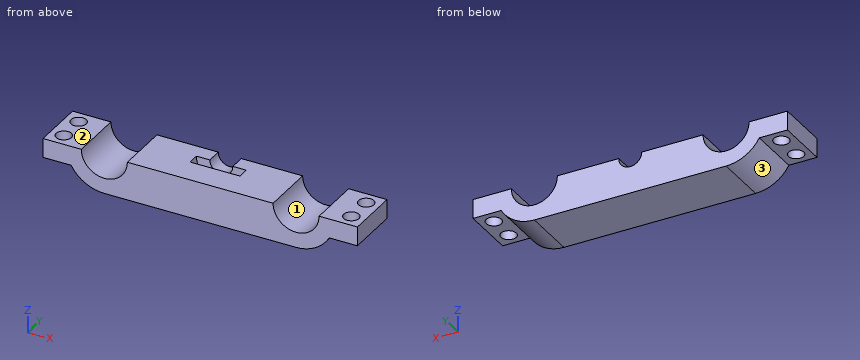
```python
from build123d import *

# Parameters (mm, degrees)
BOSS_EXTRUDE1_DEPTH     = 14
CUT_EXTRUDE1_DEPTH      = 45.463468151
CUT_EXTRUDE1_DEPTH_BACK = 45.463468151
SKETCH4_R               = 2
SKETCH5_W               = 9.30871577
SKETCH5_H               = 4.044371358
BOSS_EXTRUDE2_DEPTH     = 7
CUT_EXTRUDE2_START      = 1.5
SKETCH6_R               = 6.5
CUT_EXTRUDE2_DEPTH      = 1.5


with BuildPart() as part:
    # Sketch2 → Boss-Extrude1 (new body)
    with BuildSketch(Plane(origin=(0, 0, 0), x_dir=(1, 0, 0), z_dir=(0, 1, 0))):
        with BuildLine():
            Line((-3, 0), (-19, 0))
            ThreePointArc((-19, 0), (-25, 6), (-31, 0))
            Line((-31, 0), (-41, 0))
            Line((-41, 0), (-41, 5))
            Line((-41, 5), (-33.660254038, 5))
            ThreePointArc((-33.660254038, 5), (-30, 8.660254038), (-25, 10))
            Line((-25, 10), (25, 10))
            ThreePointArc((25, 10), (30, 8.660254038), (33.660254038, 5))
            Line((33.660254038, 5), (41, 5))
            Line((41, 5), (41, 0))
            Line((41, 0), (31, 0))
            ThreePointArc((31, 0), (25, 6), (19, 0))
            Line((19, 0), (3, 0))
            ThreePointArc((3, 0), (0, 3), (-3, 0))
        make_face()
    extrude(amount=BOSS_EXTRUDE1_DEPTH)

    # Sketch4 → Cut-Extrude1 (cut, two sides: drawn at the far end of the back side and taken through both)
    with BuildSketch(Plane.XY.offset(-CUT_EXTRUDE1_DEPTH_BACK)):
        with Locations((-37.5, 10.5)):
            Circle(SKETCH4_R)
        with Locations((-37.5, 3.5)):
            Circle(SKETCH4_R)
        with Locations((37.5, 10.5)):
            Circle(SKETCH4_R)
        with Locations((37.5, 3.5)):
            Circle(SKETCH4_R)
    extrude(amount=CUT_EXTRUDE1_DEPTH + CUT_EXTRUDE1_DEPTH_BACK, mode=Mode.SUBTRACT)

    # Sketch5 → Boss-Extrude2 (add)
    with BuildSketch(Plane.XZ):
        with Locations((-0.028958253, -2.022185679)):
            Rectangle(SKETCH5_W, SKETCH5_H)
    extrude(amount=-BOSS_EXTRUDE2_DEPTH)

    # Sketch6 → Cut-Extrude2 (cut, symmetric)
    with BuildSketch(Plane(origin=(0, 7, 0), x_dir=(1, 0, 0), z_dir=(0, 1, 0)).offset(CUT_EXTRUDE2_START)):
        Circle(SKETCH6_R)
    extrude(amount=CUT_EXTRUDE2_DEPTH, both=True, mode=Mode.SUBTRACT)


solid = part.part
```
Here's how the part is built. I have some questions about the finished solid (model axes, mm). Face numbers are marked on the shaded views. Round coordinates to 2 decimals unless told otherwise and drop trailing zeros. Order: outer loops, then holes, each group sorted by start corner. A loop starts at its lowest first (then second) coordinate and runs counter-clockwise, first axis right, second up. Notation, with made-up numbers: (-37, 87) -> (4, 87) arc R22 cw to (4, 111) -> close; hole circle Ø11 at (32, 9). An arc over 180 degrees is marked (long way). Use a Markdown table: item, result. Add a question column.
(1) If we mould it in two halves opening along X, with no side actions, what happens to the marked faces 1, 2 and 3? For each: released by +X, released by -X, zero draft, split by the parting line, or undercut.
(2) Suppose I cut it at A-A, the plane y = 3.5. Please give me the cut outline in (x, z).
(3) Suppose I cut it at D-D, the plane z = -8.5. Please give me the cut outline in (x, y), and give its area (4 significant figures).
(4) I need wall thicknesses on line 1 along Y through (x, z) = (37.5, -0.5); line 2 along Y through (x, z) = (-1, -6); line 3 along Y through (x, z) = (-36, -4). Which ranges of each line are inside material? Lowest first, please.
(5) Suppose I cut it at B-B, the plane x = -37.5. Please give me the cut outline in (y, z).
(6) Suppose I cut it at C-C, the plane x = 0. Please give me the cut outline in (y, z), and give its area (4 significant figures).
(7) For pin 1 Ø4.5 at (x, y) = (37.5, 3.5) entering from -Z; pin 2 Ø3 at (x, y) = (28.5, 1.5) entering from -Z; pin 3 Ø1.5 at (y, z) = (4, -6.5) entering from +X, each with a flat end and sliding along its axis, tell me the tip position at first contact or that it passes through.
Verdict:
| question | item | result |
|---|---|---|
| 1 | face 1 | undercut |
| 1 | face 2 | zero draft |
| 1 | face 3 | released by -X |
| 2 | outline | (-41, -5) -> (-39.5, -5) -> (-39.5, 0) -> (-41, 0) -> close; (-35.5, -5) -> (-33.66, -5) arc R10 ccw to (-25, -10) -> (25, -10) arc R10 ccw to (33.66, -5) -> (35.5, -5) -> (35.5, 0) -> (31, 0) arc R6 cw to (19, 0) -> (-19, 0) arc R6 cw to (-31, 0) -> (-35.5, 0) -> close; (39.5, -5) -> (41, -5) -> (41, 0) -> (39.5, 0) -> close |
| 3 | outline | (-30.27, 0) -> (30.27, 0) -> (30.27, 14) -> (-30.27, 14) -> close |
| 3 | area | 847.5 mm2 |
| 4 | line 1 | 0 to 1.5, 5.5 to 8.5, 12.5 to 14 |
| 4 | line 2 | 0 to 7, 10 to 14 |
| 4 | line 3 | 0 to 2.18, 4.82 to 9.18, 11.82 to 14 |
| 5 | outline | (0, -5) -> (1.5, -5) -> (1.5, 0) -> (0, 0) -> close; (5.5, -5) -> (8.5, -5) -> (8.5, 0) -> (5.5, 0) -> close; (12.5, -5) -> (14, -5) -> (14, 0) -> (12.5, 0) -> close |
| 6 | outline | (0, -10) -> (14, -10) -> (14, -3) -> (10, -3) -> (10, -6.5) -> (7, -6.5) -> (7, 0) -> (0, 0) -> close |
| 6 | area | 108.5 mm2 |
| 7 | pin 1 | z = -5 |
| 7 | pin 2 | z = -9.8 |
| 7 | pin 3 | x = 33.18 |
